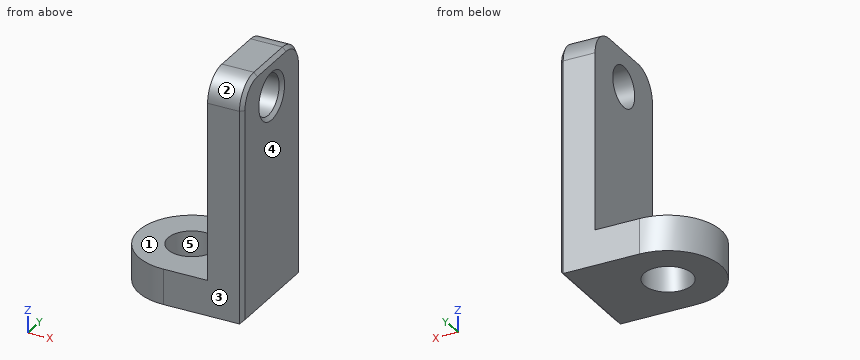
from build123d import *

# Parameters (mm, degrees)
F0_R     = 1.35
F1_W     = 2
F1_H     = 6
F5_R     = 1.15
F6_DEPTH = 17.001
F7_R     = 1.5
F8_SIZE  = 0.2


with BuildPart() as f3:
    # F3: sweep along a path in F2
    with BuildLine(Plane.XZ) as f3_path:
        Line((0, -2), (0, 0))
    # F0 (on Top) → F3 (sweep)
    with BuildSketch(Plane.XY):
        with BuildLine():
            Line((-9.5, -3), (-9.5, 3))
            Line((-9.5, 3), (-14, 3))
            ThreePointArc((-14, 3), (-17, 0), (-14, -3))
            Line((-14, -3), (-9.5, -3))
        make_face()
        with Locations((-14, 0)):
            Circle(F0_R, mode=Mode.SUBTRACT)
    sweep(path=f3_path.line)

    # F4: sweep along a path in F2
    with BuildLine(Plane.XZ) as f4_path:
        Line((0, 0), (0, 11.5))
    # F1 (on Top) → F4 (sweep)
    with BuildSketch(Plane.XY):
        with Locations((-10.5, 0)):
            Rectangle(F1_W, F1_H)
    sweep(path=f4_path.line)

    # F5 (on Right) → F6 (cut, through all)
    with BuildSketch(Plane.YZ):
        with Locations((0, 9.5)):
            Circle(F5_R)
    extrude(amount=-F6_DEPTH, mode=Mode.SUBTRACT)

    # F7
    f7_edges = [f3.edges().sort_by_distance(p)[0] for p in [
        (-10.5, 3, 11.5),
        (-10.5, -3, 11.5),
    ]]
    fillet(f7_edges, radius=F7_R)

    # F8
    f8_edges = [f3.edges().sort_by_distance(p)[0] for p in [
        (-9.5, -3, 4),
        (-9.5, -2.56066, 11.06066),
        (-9.5, 0, -2),
        (-9.5, 0, 11.5),
        (-9.5, 3, 4),
        (-9.5, 2.56066, 11.06066),
        (-9.5, -1.15, 9.5),
    ]]
    chamfer(f8_edges, length=F8_SIZE)


solid = f3.part
The model under review builds one solid part; all positions refer to its coordinate system, in mm. Face numbers are marked on the shaded views. A direction names the side the tool comes from. Give positions to 0.01 mm unless a question says otherwise; leave off trailing zeros. Order: outer loops, then holes, each group sorted by start corner. A loop starts at its lowest first (then second) coordinate and runs counter-clockwise, first axis right, second up. Notation, with made-up numbers: (18.5, 84) -> (47.5, 84) arc R13 cw to (47.5, 101) -> close; hole circle Ø1 at (-20, 29.25). An arc over 180 degrees is marked (long way). Write item = value, one per line. Start each with the question number.
(1) For L1, parallel to Y at x = -14, z = -1.05; L2, parallel to Z at x = -10.7, y = 0; L3, parallel to X at y = 0.9, z = 1, list the stretches that pass through material, from the lowest coordinate up. Write a range as from..to.
(2) Tool access review of the marked faces 1 and 2: name each direction out of +Z, -Z, +X, -X, +Y, -Y from which nothing blocks a thin tool from reaching the whole face with its end or side.
(3) Take a section at B-B (x = -10.5). Write out the cut boundary in (y, z), plus the area to 3 significant figures.
(4) Draft analysis for pull direction Y (two halves, no side actions). For the marked faces 3, 4 and 5, state which applies: +Y half, -Y half, draft (parallel to the pull), parting line (faces both ways), or undercut.
(5) Take a section at D-D (x = -13). Write out the cut boundary in (y, z), plus the area to 3 significant figures.
(6) Take a section at A-A (z = 9.5). Write out the cut boundary in (x, y).
(7) For pin 1 Ø3 at (x, y) = (-13.5, 0.5) entering from +Z; pin 2 Ø2 at (y, z) = (0, 9.5) entering from -X; pin 3 Ø3 at (y, z) = (0, 3.5) entering from -X, all flat-tipped, find the tip position at first contact; note any pin that passes through.
(8) Take a section at C-C (y = 0). Write out the cut boundary in (x, z).
Returned:
q1.L1 = -3..-1.35, 1.35..3
q1.L2 = -2..8.35, 10.65..11.5
q1.L3 = -11.5..-9.5
q2.face_1 = +Z, -X, +Y, -Y
q2.face_2 = +Z, +X, -X, -Y
q3.outline = (-3, -2) -> (3, -2) -> (3, 10) arc R1.5 ccw to (1.5, 11.5) -> (-1.5, 11.5) arc R1.5 ccw to (-3, 10) -> close; hole circle Ø2.3 at (0, 9.5)
q3.area = 75.9 mm²
q4.face_3 = -Y half
q4.face_4 = draft
q4.face_5 = undercut
q5.outline = (-3, -2) -> (-0.91, -2) -> (-0.91, 0) -> (-3, 0) -> close; (0.91, -2) -> (3, -2) -> (3, 0) -> (0.91, 0) -> close
q5.area = 8.37 mm²
q6.outline = (-11.5, -3) -> (-9.7, -3) -> (-9.5, -2.8) -> (-9.5, -1.35) -> (-9.7, -1.15) -> (-11.5, -1.15) -> close; (-11.5, 1.15) -> (-9.7, 1.15) -> (-9.5, 1.35) -> (-9.5, 2.8) -> (-9.7, 3) -> (-11.5, 3) -> close
q7.pin_1 = 0
q7.pin_2 = through
q7.pin_3 = -11.5
q8.outline = (-17, -2) -> (-15.35, -2) -> (-15.35, 0) -> (-17, 0) -> close; (-12.65, -2) -> (-9.7, -2) -> (-9.5, -1.8) -> (-9.5, 8.15) -> (-9.7, 8.35) -> (-11.5, 8.35) -> (-11.5, 0) -> (-12.65, 0) -> close; (-11.5, 10.65) -> (-9.7, 10.65) -> (-9.5, 10.85) -> (-9.5, 11.3) -> (-9.7, 11.5) -> (-11.5, 11.5) -> close
